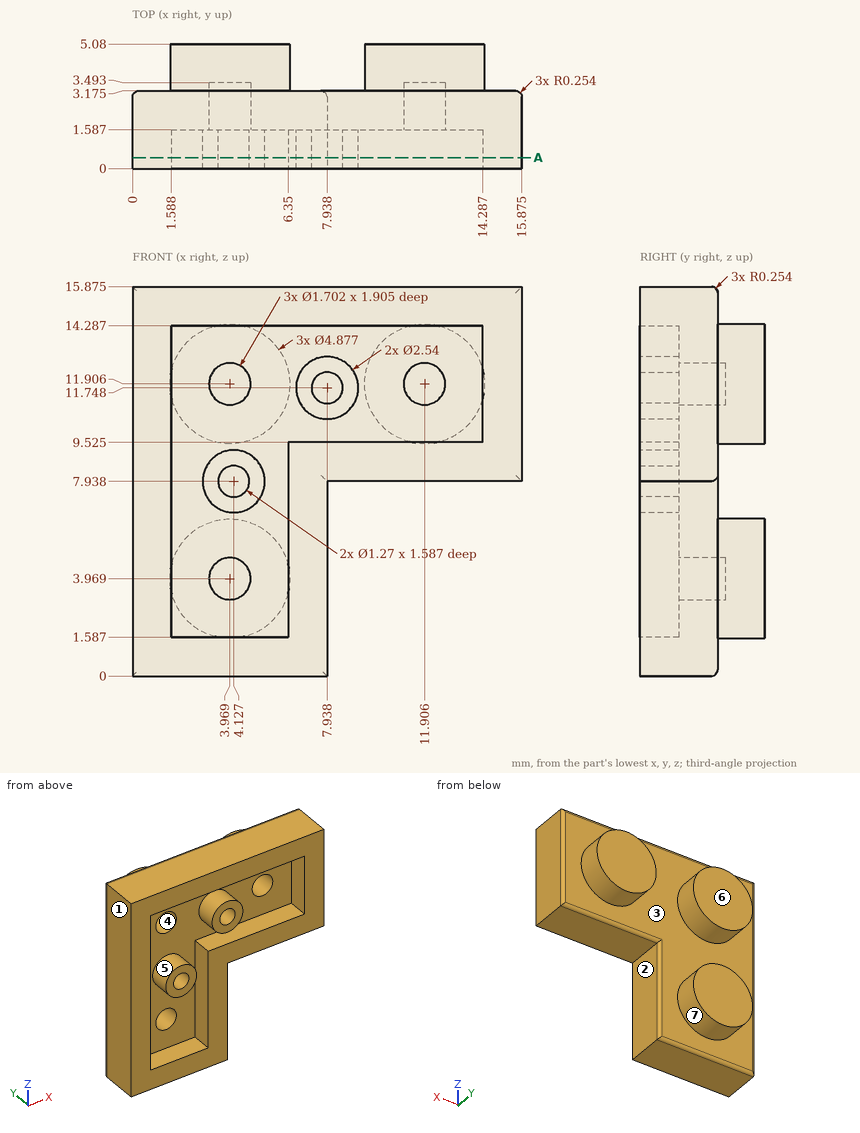
For this review, use the dimensioned drawing (mm, ordinates from the lowest corner) and the shaded views. A direction names the side the tool comes from. Round coordinates to 2 decimals unless told otherwise and drop trailing zeros. Write each question's results on one line, items separated by ' | '. Start each with the question number.
1. Clearance check with flat-ended pins moving along their axes: pin 1 Ø1 at (y, z) = (1.5, 2) entering from +X; pin 2 Ø1.5 at (x, y) = (11.5, 2) entering from -Z; pin 3 Ø0.5 at (x, z) = (4.5, 12) entering from -Y. State where each tip first meets the part, or that it passes through.
2. Draft analysis for pull direction X (two halves, no side actions). For the marked faces 5, 6 and 7, state which applies: pulls with the +X half, pulls with the -X half, needs draft (parallel to the pull), parting line crosses it, or undercut.
3. Tool access review of the marked faces 1, 2, 3 and 4: name each direction out of +Z, -Z, +X, -X, +Y, -Y from which nothing blocks a thin tool from reaching the whole face with its end or side.
4. Add section A-A (y = 0.45). State how many separate pieces and enclosed holes the cut face has.
5. To check wall thickness, follow L1, parallel to X at y = 3.35, z = 4; L2, parallel to Z at x = 7, y = 0.35 (1 decimal); L3, parallel to X at y = 0.6, z = 6. State the ranges of each line that lie inside material, in increasing order. Write a range as [from, to].
Output values:
1) pin 1: x = 7.94 | pin 2: z = 7.94 | pin 3: y = 3.49
2) face 5: undercut | face 6: needs draft | face 7: parting line crosses it
3) face 1: +Z, -Z, -X, +Y, -Y | face 2: -Z, +X, +Y, -Y | face 3: +Y | face 4: -Y
4) separate pieces: 3 | enclosed holes: 3
5) L1: [1.53, 3.12], [4.82, 6.41] | L2: [0, 9.5], [10.9, 12.6], [14.3, 15.9] | L3: [0, 1.59], [6.35, 7.94]
